Autodesk Inventor part; units mm, degrees
ref_plane "YZ Plane" through (0, 0, 0) normal (1, 0, 0) x (0, 1, 0)
ref_plane "XZ Plane" through (0, 0, 0) normal (0, 1, 0) x (-1, 0, 0)
ref_plane "XY Plane" through (0, 0, 0) normal (0, 0, 1) x (1, 0, 0)
sketch "Sketch1" plane through (0, 0, 0) normal (0, 0, 1) x (1, 0, 0)
  line L0 (-7.619, -8.598) -> (7.601, -8.598)
  line L1 (7.601, -8.598) -> (7.601, 10.452)
  line L2 (7.601, 10.452) -> (-7.619, 10.452)
  line L3 (-7.619, 10.452) -> (-7.619, -8.598)
  line L4 (-6.394, 9.217) -> (6.376, 9.217)
  line L5 (6.376, 9.217) -> (6.376, -7.363)
  line L6 (6.376, -7.363) -> (-6.394, -7.363)
  line L7 (-6.394, -7.363) -> (-6.394, 9.217)
  circle A0 centre (-6.394, 9.217) radius 0.58
  circle A1 centre (6.376, 9.217) radius 0.58
  circle A2 centre (6.376, -7.363) radius 0.58
  circle A3 centre (-6.394, -7.363) radius 0.58
  line L8 (-3.844, -9.748) -> (3.826, -9.748)
  line L9 (3.826, -9.748) -> (3.826, -8.598)
  line L10 (-3.844, -9.748) -> (-3.844, -8.598)
  line L11 (5.796, 8.637) -> (-5.814, 8.637)
  line L12 (-5.814, 8.637) -> (-5.814, -2.973)
  line L13 (-5.814, -2.973) -> (5.796, -2.973)
  line L14 (5.796, -2.973) -> (5.796, 8.637)
  line L15 (3.826, -9.748) -> (-3.844, -9.748)
  line L16 (-3.844, -9.748) -> (-3.844, -4.118)
  line L17 (-3.844, -4.118) -> (3.826, -4.118)
  line L18 (3.826, -4.118) -> (3.826, -9.748)
  line L19 (-6.394, -6.203) -> (-4.894, -6.203)
  line L20 (-4.894, -6.203) -> (-4.894, -3.703)
  line L21 (-4.894, -3.703) -> (-6.394, -3.703)
  line L22 (-6.394, -3.703) -> (-6.394, -6.203)
  line L23 (-7.619, 8.057) -> (-6.394, 8.057)
  line L24 (-6.394, 8.057) -> (-6.394, -6.783)
  line L25 (-7.619, -6.783) -> (-7.619, 8.057)
  line L26 (7.601, 8.637) -> (7.601, -6.783)
  line L27 (6.376, -6.783) -> (6.376, 8.637)
  line L28 (-6.394, 10.452) -> (-6.394, 9.797)
  line L29 (6.376, 10.452) -> (6.376, 9.797)
  line L30 (-7.619, -6.203) -> (-6.394, -6.203)
  line L31 (6.376, -6.203) -> (7.601, -6.203)
  line L32 (6.376, 8.057) -> (7.601, 8.057)
  point P0 (0, 0)
  point P1 (2.2173, 6.5337)
  point P2 (-0.009, -8.598)
  point P3 (-0.009, -9.748)
  point P4 (-6.394, -3.703)
  point P5 (-4.894, -4.953)
  point P6 (-5.644, -6.203)
  point P7 (-6.394, 8.057)
  point P8 (-7.0065, -6.783)
  point P9 (6.9885, 8.637)
  point P10 (-7.0065, -6.203)
  dimension "d16" = 1.16
  dimension "d17" = 1.16
  dimension "d0" = 15.22
  dimension "d1" = 19.05
  dimension "d14" = 12.77
  dimension "d15" = 16.58
  dimension "d18" = 1.16
  dimension "d19" = 1.16
  dimension "d23" = 1.235
  dimension "d24" = 1.225
  dimension "d47" = 1.15
  dimension "d55" = 5.63
  dimension "d60" = 1.5
  dimension "d61" = 2.5
  dimension "d64" = 2.395
  dimension "d67" = 2.395
extrude "Extrusion1" add sketch "Sketch1" against normal blind 2 contours L3 L30 L7 A3 L6 L16 L0 | L16 L6 L18 L0 | L18 L6 A2 L5 L31 L1 L0 | L16 L17 L18 L6 | L6 A3 L7 L19 L20 L21 A0 L4 A1 L5 A2 L18 L17 L16 | L3 L23 L7 L30 | L3 L2 L28 A0 L7 L23 | L7 L21 L20 L19 | L31 L5 L32 L1 | L2 L29 A1 L4 A0 L28 | L32 L5 A1 L29 L2 L1 | L14 L13 L12 L11
extrude "Extrusion6" add sketch "Sketch1" along normal blind 5 contours L14 L13 L12 L11
extrude "Extrusion7" add sketch "Sketch1" along normal blind 2.95 contours L16 L6 L18 L0 | L0 L9 L8 L10 | L16 L17 L18 L6
extrude "Extrusion8" add sketch "Sketch1" along normal blind 1.5 contours L7 L21 L20 L19
extrude "Extrusion10" cut sketch "Sketch1" against normal blind 2 contours L3 L23 L7 L30 | L31 L5 L32 L1
fillet "Fillet13" radius 1.22 12 edges at (7.601, 10.452, -1) (7.601, 8.057, -1) (6.376, 8.057, -1) (7.601, -6.203, -1) (6.376, -6.203, -1) (7.601, -8.598, -1) (-6.394, -6.203, -1) (-7.619, -6.203, -1) (-7.619, -8.598, -1) (-7.619, 10.452, -1) (-7.619, 8.057, -1) (-6.394, 8.057, -1)
properties part number "IR_cam"
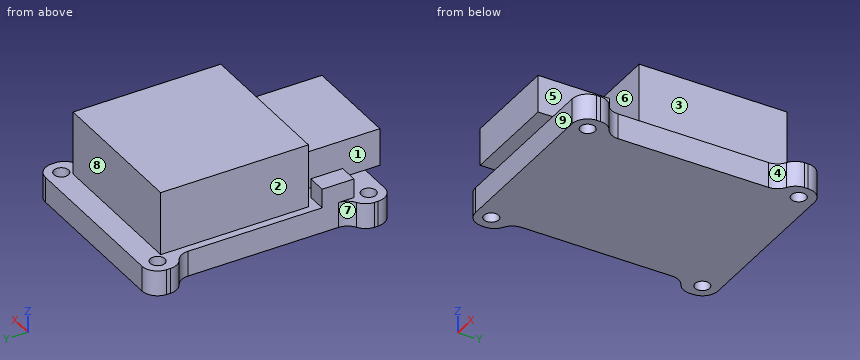
Input: part model. Units: mm. Frame: model coordinates. Face numbers are marked on the shaded views. A direction names the side the tool comes from. Coordinates: 2 decimals unless noted, no trailing zeros. Loops run counter-clockwise (first coordinate to the right, second up) from the corner with the lowest first, then second, coordinate; pieces in that order, holes last. Notation, with made-up numbers: (-6.5, 41.25) -> (15.5, 41.25) arc R32 ccw to (15.5, 67.25) -> close; hole circle Ø4 at (47, 69). An arc over 180 degrees is marked (long way). Write each question's results on one line, items separated by ' | '. Start each with the question number.
Q1. Reachability of the marked faces 1, 2, 3, 4 and 5 from +Z, -Z, +X, -X, +Y, -Y: full face, straight path, thin tool, end or side. Return the list, or none.
Q2. Ray query, line 1 (Y direction, x = -1.75, z = 0.75); line 2 (Y direction, x = -5.25, z = 0.75); line 3 (Z direction, x = 4, y = -8). Return the intervals inside material, ascending. Write a range as from..to.
Q3. Pull-direction query (Y, two-part tool) for the marked faces 6, 7, 8 and 9; classes: released by +Y, released by -Y, zero draft, split by the parting line, or undercut.
Q4. Section B-B, the plane x = -0.5. Return the cut outline in (y, z).
Q5. Section D-D, the plane y = 5.5. Return the cut outline in (x, z), plus the area to 3 significant figures.
Q6. Section C-C, the plane z = 0.25. Return the cut outline in (x, y), plus the area to 3 significant figures.
Q7. Pin query (flat end, axial travel): pin 1 (0.9 mm diameter, centred on y = -7.5, z = 2, fed in from -X); pin 2 (1 mm diameter, centred on y = 1.5, z = -1, fed in from -X); pin 3 (1.6 mm diameter, centred on x = -5.5, z = 1, fed in from -Y); pin 4 (3 mm diameter, centred on x = -2.5, z = 3.5, fed in from -Y). Return the tip coordinate at first contact, or that it passes through.
Q8. Section A-A, the plane z = 2.5. Return the cut outline in (x, y).
Found:
1) face 1: +Z, -Y | face 2: +Z, -X, +Y | face 3: +Z, +X, +Y, -Y | face 4: +Z, -Z, +X | face 5: +Z, +X, -Y
2) line 1: -9.75..-4.12, -2.97..8.64 | line 2: -6.2..-3.7, -2.97..8.64 | line 3: -2..0
3) face 6: undercut | face 7: undercut | face 8: released by +Y | face 9: released by -Y
4) outline: (-9.75, 0) -> (-8.6, 0) -> (-8.6, -2) -> (10.45, -2) -> (10.45, 0) -> (8.64, 0) -> (8.64, 5) -> (-2.97, 5) -> (-2.97, 0) -> (-4.12, 0) -> (-4.12, 2.95) -> (-9.75, 2.95) -> close
5) outline: (-6.39, -2) -> (6.38, -2) -> (6.38, 0) -> (5.8, 0) -> (5.8, 5) -> (-5.81, 5) -> (-5.81, 0) -> (-6.39, 0) -> close | area: 83.6 mm2
6) outline: (-6.39, -6.2) -> (-4.89, -6.2) -> (-4.89, -3.7) -> (-6.39, -3.7) -> close; (-5.81, -2.97) -> (5.8, -2.97) -> (5.8, 8.64) -> (-5.81, 8.64) -> close; (-3.84, -9.75) -> (3.83, -9.75) -> (3.83, -4.12) -> (-3.84, -4.12) -> close | area: 182 mm2
7) pin 1: x = -3.84 | pin 2: x = -6.39 | pin 3: y = -6.2 | pin 4: y = -9.75
8) outline: (-5.81, -2.97) -> (5.8, -2.97) -> (5.8, 8.64) -> (-5.81, 8.64) -> close; (-3.84, -9.75) -> (3.83, -9.75) -> (3.83, -4.12) -> (-3.84, -4.12) -> close
